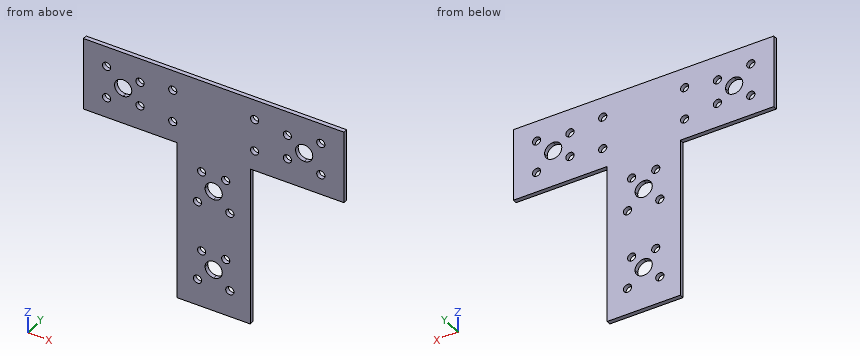
from build123d import *

# Parameters (mm, degrees)
F1_DEPTH = 2.61
F2_R     = 2.5
F3_DEPTH = 2.611


with BuildPart() as f1:
    # F0 (on Front) → F1 (new body)
    with BuildSketch(Plane.XZ):
        Polygon((79.5, -22.52), (79.5, 22.52), (-79.5, 22.52), (-79.5, -22.52), (-22.35, -22.52), (-22.35, -121.48), (22.35, -121.48), (22.35, -22.52), align=None)
        with BuildLine():
            ThreePointArc((0, -89.98), (3.712311, -91.517689), (5.25, -95.23))
            ThreePointArc((5.25, -95.23), (3.712311, -98.942311), (0, -100.48))
            ThreePointArc((0, -100.48), (-3.712311, -98.942311), (-5.25, -95.23))
            ThreePointArc((-5.25, -95.23), (-3.712311, -91.517689), (0, -89.98))
        make_face(mode=Mode.SUBTRACT)
        with BuildLine():
            ThreePointArc((-55.25, 5.25), (-51.537689, 3.712311), (-50, 0))
            ThreePointArc((-50, 0), (-51.537689, -3.712311), (-55.25, -5.25))
            ThreePointArc((-55.25, -5.25), (-60.5, 0), (-55.25, 5.25))
        make_face(mode=Mode.SUBTRACT)
        with BuildLine():
            ThreePointArc((-5.25, -45.23), (-3.712311, -41.517689), (0, -39.98))
            ThreePointArc((0, -39.98), (3.712311, -41.517689), (5.25, -45.23))
            ThreePointArc((5.25, -45.23), (3.712311, -48.942311), (0, -50.48))
            ThreePointArc((0, -50.48), (-3.712311, -48.942311), (-5.25, -45.23))
        make_face(mode=Mode.SUBTRACT)
        with BuildLine():
            ThreePointArc((55.25, 5.25), (58.962311, 3.712311), (60.5, 0))
            ThreePointArc((60.5, 0), (58.962311, -3.712311), (55.25, -5.25))
            ThreePointArc((55.25, -5.25), (50, 0), (55.25, 5.25))
        make_face(mode=Mode.SUBTRACT)
    extrude(amount=F1_DEPTH)

    # F2 (on face) → F3 (cut, through all)
    with BuildSketch(Plane.XZ.offset(2.61)):
        with Locations((65.4, 10.02)):
            Circle(F2_R)
        with Locations((65.4, -10.02)):
            Circle(F2_R)
        with Locations((45, 7.52)):
            Circle(F2_R)
        with Locations((45, -7.52)):
            Circle(F2_R)
        with Locations((25, 10.02)):
            Circle(F2_R)
        with Locations((25, -10.02)):
            Circle(F2_R)
        with Locations((-25, 10.02)):
            Circle(F2_R)
        with Locations((-25, -10.02)):
            Circle(F2_R)
        with Locations((-45, 7.52)):
            Circle(F2_R)
        with Locations((-45, -7.52)):
            Circle(F2_R)
        with Locations((-65.4, -10.02)):
            Circle(F2_R)
        with Locations((-65.4, 10.02)):
            Circle(F2_R)
        with Locations((9.85, -55.48)):
            Circle(F2_R)
        with Locations((-9.85, -55.48)):
            Circle(F2_R)
        with Locations((-9.85, -104.98)):
            Circle(F2_R)
        with Locations((9.85, -104.98)):
            Circle(F2_R)
        with Locations((-7.35, -35.48)):
            Circle(F2_R)
        with Locations((7.35, -35.48)):
            Circle(F2_R)
        with Locations((7.35, -85.98)):
            Circle(F2_R)
        with Locations((-7.35, -85.98)):
            Circle(F2_R)
    extrude(amount=-F3_DEPTH, mode=Mode.SUBTRACT)


solid = f1.part
CAD build for the part. Positions are in the model's coordinates, mm. Give positions to 0.01 mm unless a question says otherwise; leave off trailing zeros. Order: outer loops, then holes, each group sorted by start corner. A loop starts at its lowest first (then second) coordinate and runs counter-clockwise, first axis right, second up. Notation, with made-up numbers: (-15.75, 31.25) - (32.25, 31.25) arc R4 ccw to (32.25, 38.25) - close; hole circle Ø8 at (-18.5, 62). An arc over 180 degrees is marked (long way). Answer in a Markdown table with one row per item.
1. Saw through at D-D, the plane z = -28. Give the cut face in (x, y).
Data:
| item | result |
|---|---|
| outline | (-22.35, -2.61) - (22.35, -2.61) - (22.35, 0) - (-22.35, 0) - close |
2. Saw through at C-C, the plane y = -0.9. Count the separate pieces of the cut face and the enclosed holes in it, plus the area to 3 significant figures.
Data:
| item | result |
|---|---|
| separate pieces | 1 |
| enclosed holes | 24 |
| area | 10,800 mm² |
3. Flat gauge pins, fed straight in: pin 1 (1.5 mm diameter, centred on x = 37, y = -0.5, fed in from -Z); pin 2 (1.3 mm diameter, centred on y = -1.5, z = -76.5, fed in from +X). Where does each tip first touch, or does it go through?
Data:
| item | result |
|---|---|
| pin 1 | stops at z = -22.52 |
| pin 2 | stops at x = 22.35 |
4. Probe probe 1 along Z at (x, y) = (-65.4, -1.05); probe 2 along Z at (x, y) = (46, -1.6); probe 3 along X at (y, z) = (-0.45, 2.5). List the from-to ranges inside material, lowest first. Write a range as [from, to].
Data:
| item | result |
|---|---|
| probe 1 | z = [-22.52, -12.52], [-7.52, 7.52], [12.52, 22.52] |
| probe 2 | z = [-22.52, -9.81], [-5.23, 5.23], [9.81, 22.52] |
| probe 3 | x = [-79.5, -59.87], [-50.63, 50.63], [59.87, 79.5] |
5. Saw through at A-A, the plane z = -55.48. Give the cut face in (x, y).
Data:
| item | result |
|---|---|
| outline | (-22.35, -2.61) - (-12.35, -2.61) - (-12.35, 0) - (-22.35, 0) - close; (-7.35, -2.61) - (7.35, -2.61) - (7.35, 0) - (-7.35, 0) - close; (12.35, -2.61) - (22.35, -2.61) - (22.35, 0) - (12.35, 0) - close |
6. Saw through at B-B, the plane x = -25. Give the cut face in (y, z).
Data:
| item | result |
|---|---|
| outline | (-2.61, -22.52) - (0, -22.52) - (0, -12.52) - (-2.61, -12.52) - close; (-2.61, -7.52) - (0, -7.52) - (0, 7.52) - (-2.61, 7.52) - close; (-2.61, 12.52) - (0, 12.52) - (0, 22.52) - (-2.61, 22.52) - close |
